Check sheet for the modelled part. Datum: model origin and axes. Units: mm. A direction names the side the tool comes from. Coordinates: 2 decimals unless noted, no trailing zeros. Write each loop counter-clockwise with the first axis right and the second up, starting at its lowest first coordinate (ties: lowest second). Pieces come first, ordered by that corner, then holes. Notation, with made-up numbers: (0, 89) - (37, 89) arc R7 ccw to (37, 98) - close; hole circle Ø6 at (32, -18). An arc over 180 degrees is marked (long way). Write each question's results on one line, items separated by ' | '.
from build123d import *

# Parameters (mm, degrees)
SKETCH_1_R          = 8.5
EXTRUDE_1_DEPTH     = 2.5
SKETCH_2_R          = 9.5
EXTRUDE_2_DEPTH     = 3.4
SKETCH_3_R          = 1.1
CUT_EXTRUDE_1_DEPTH = 15.673445403


with BuildPart() as part:
    # ｽｹｯﾁ1 → ﾎﾞｽ - 押し出し1 (new body)
    with BuildSketch(Plane.XY):
        Circle(SKETCH_1_R)
    extrude(amount=EXTRUDE_1_DEPTH)

    # ｽｹｯﾁ2 → ﾎﾞｽ - 押し出し2 (add)
    with BuildSketch(Plane.XY.offset(2.5)):
        Circle(SKETCH_2_R)
    extrude(amount=EXTRUDE_2_DEPTH)

    # ｽｹｯﾁ3 → ｶｯﾄ - 押し出し1 (cut, through all)
    with BuildSketch(Plane(origin=(0, 0, 0), x_dir=(-1, 0, 0), z_dir=(0, 0, -1))):
        with Locations((0, 6)):
            Circle(SKETCH_3_R)
        with Locations((5.196152423, -3)):
            Circle(SKETCH_3_R)
        with Locations((-5.196152423, -3)):
            Circle(SKETCH_3_R)
    extrude(amount=-CUT_EXTRUDE_1_DEPTH, mode=Mode.SUBTRACT)


solid = part.part
1. Material ranges on L1, parallel to Y at x = 0, z = 3.4; L2, parallel to X at y = 5, z = 4; L3, parallel to Y at x = 0, z = 1.9, recorded low to high. Write a range as [from, to].
Values follow:
L1: y = [-9.5, 4.9], [7.1, 9.5] | L2: x = [-8.08, -0.46], [0.46, 8.08] | L3: y = [-8.5, 4.9], [7.1, 8.5]
2. Sectioned sample at D-D (y = -3). Record the cut outline in (x, z), then the cut area to 3 significant figures.
Values follow:
outline: (-9.01, 2.5) - (-7.95, 2.5) - (-7.95, 0) - (-6.3, 0) - (-6.3, 5.9) - (-9.01, 5.9) - close; (-4.1, 0) - (4.1, 0) - (4.1, 5.9) - (-4.1, 5.9) - close; (6.3, 0) - (7.95, 0) - (7.95, 2.5) - (9.01, 2.5) - (9.01, 5.9) - (6.3, 5.9) - close | area: 75.1 mm^2
3. Sectioned sample at C-C (z = 1.1). Record the cut outline in (x, y), then the cut area to 3 significant figures.
Values follow:
outline: circle Ø17 at (0, 0); hole circle Ø2.2 at (-5.2, -3); hole circle Ø2.2 at (0, 6); hole circle Ø2.2 at (5.2, -3) | area: 216 mm^2
4. Sectioned sample at B-B (y = 0). Record the cut outline in (x, z).
Values follow:
outline: (-9.5, 2.5) - (-8.5, 2.5) - (-8.5, 0) - (8.5, 0) - (8.5, 2.5) - (9.5, 2.5) - (9.5, 5.9) - (-9.5, 5.9) - close
5. Draft check along X on faces 3 (the flat face through (0, 0, 0)), 4 (the cylindrical face through (4.38, -8.43, 4.18)), 5 (the cylindrical face through (-0.59, 6.93, 2.91)). Enter one of: pulls with the +X half, pulls with the -X half, needs draft (parallel to the pull), parting line crosses it, or undercut.
Values follow:
face 3: needs draft | face 4: parting line crosses it | face 5: undercut
6. Sectioned sample at A-A (x = 0). Record the cut outline in (y, z), then the cut area to 3 significant figures.
Values follow:
outline: (-9.5, 2.5) - (-8.5, 2.5) - (-8.5, 0) - (4.9, 0) - (4.9, 5.9) - (-9.5, 5.9) - close; (7.1, 0) - (8.5, 0) - (8.5, 2.5) - (9.5, 2.5) - (9.5, 5.9) - (7.1, 5.9) - close | area: 94.1 mm^2
7. Access from +Z, -Z, +X, -X, +Y, -Y to the whole of each face (thin tool, end or side, straight path). Record for faces 1 (the cylindrical face through (4.57, 7.167, 1.232)), 2 (the cylindrical face through (4.147, -2.67, 2.909)).
Values follow:
face 1: -Z | face 2: +Z, -Z
8. Go/stop test with a flat-tipped pin: pin 1 (1.8 mm diameter, centred on x = 5.2, y = -3, fed in from +Z). Record where the tip stops, or that it passes through.
Values follow:
pin 1: passes through
